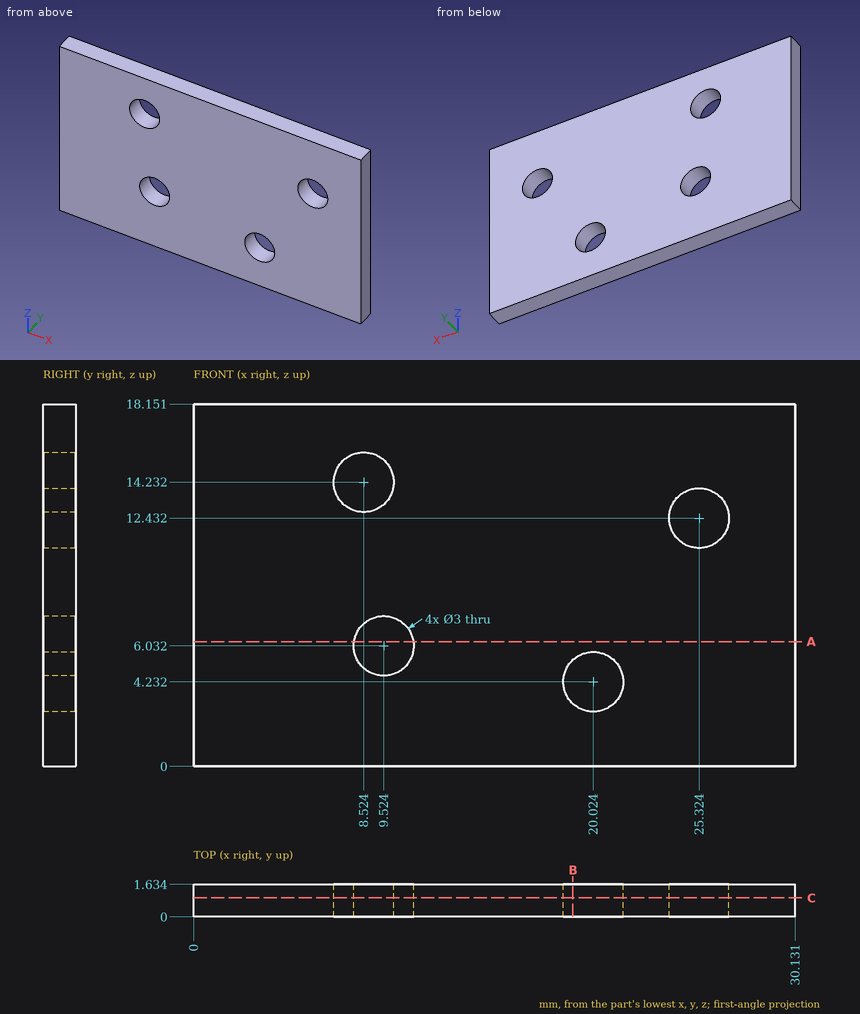
Could you check a few things on this drawing? It's one solid part, dimensions in mm from its lowest x, y, z. Round coordinates to 2 decimals unless told otherwise and drop trailing zeros. Loops run counter-clockwise (first coordinate to the right, second up) from the corner with the lowest first, then second, coordinate; pieces in that order, holes last. Notation, with made-up numbers: (1.5, -23.5) -> (13.5, -23.5) arc R27 cw to (13.5, 12.5) -> close; hole circle Ø7 at (15, 22.5). An arc over 180 degrees is marked (long way). One line per item, written item: value. Start each with the question number.
1. If we section it at C-C, the plane y = 0.95: Write out the boundary of the cut face in (x, z).
2. If we section it at A-A, the plane z = 6.25: Write out the boundary of the cut face in (x, y).
3. If we section it at B-B, the plane x = 19: Write out the boundary of the cut face in (y, z) (1 decimal).
4. If I drill on probe 1 along X at (y, z) = (1.45, 4.25); probe 2 along Z at (x, y) = (20, 1.4); probe 3 along X at (y, z) = (1.6, 5.5) (1 decimal), over which ranges is the centre line in solid material (lowest first)?
Calculated:
1. outline: (0, 0) -> (30.13, 0) -> (30.13, 18.15) -> (0, 18.15) -> close; hole circle Ø3 at (8.52, 14.23); hole circle Ø3 at (9.52, 6.03); hole circle Ø3 at (20.02, 4.23); hole circle Ø3 at (25.32, 12.43)
2. outline: (0, 0) -> (8.04, 0) -> (8.04, 1.63) -> (0, 1.63) -> close; (11.01, 0) -> (30.13, 0) -> (30.13, 1.63) -> (11.01, 1.63) -> close
3. outline: (0, 0) -> (1.6, 0) -> (1.6, 3.1) -> (0, 3.1) -> close; (0, 5.3) -> (1.6, 5.3) -> (1.6, 18.2) -> (0, 18.2) -> close
4. probe 1: x = 0 to 18.52, 21.52 to 30.13
4. probe 2: z = 0 to 2.73, 5.73 to 18.15
4. probe 3: x = 0 to 8.1, 10.9 to 19.2, 20.8 to 30.1
